For this review, take the finished solid that the model builds, in its own axes (mm). Face numbers are marked on the shaded views. A direction names the side the tool comes from. Coordinates: 2 decimals unless noted, no trailing zeros. Write each loop counter-clockwise with the first axis right and the second up, starting at its lowest first coordinate (ties: lowest second). Pieces come first, ordered by that corner, then holes. Notation, with made-up numbers: (-32, 7) - (-2, 7) arc R14 cw to (-2, 11) - close; hole circle Ø9 at (45, -32.5). An arc over 180 degrees is marked (long way). Use one line per item in the form item = value. Start each with the question number.
1) Tool access review of the marked faces 1, 2 and 3: name each direction out of +Z, -Z, +X, -X, +Y, -Y from which nothing blocks a thin tool from reaching the whole face with its end or side.
2) We need section C-C (y = 21.5). Give the boundary of the cut face in (x, z), plus the area to 3 significant figures.
3) We need section A-A (z = 3). Count the separate pieces of the cut face and the enclosed holes in it, plus the area to 3 significant figures.
4) For L1, parallel to Y at x = 23, z = 13.25; L2, parallel to Z at x = -52.5, y = -3, list the stretches that pass through material, from the lowest coordinate up. Write a range as from..to.
5) We need section B-B (x = -44.5). Give the boundary of the cut face in (y, z).
6) Insertion check: P1, Ø11.5, axis at x = 56, z = 9, coming from the -Y side; P2, Ø4.5, axis at x = -5.5, z = 6.5, coming from the +Y side; P3, Ø9.5, axis at y = 14, z = 7, coming from the -X side. Each pin has a flat end and moves straight along its axis. Give the tip position at first contact, or say it passes through.
```python
from build123d import *

# Parameters (mm, degrees)
F0_W     = 138
F0_H     = 55.5
F1_DEPTH = 1.5875
F2_W     = 14.4751365056
F2_H     = 21.9978075475
F3_DEPTH = 19


# Not quite as in the source:
# - a feature names something its author has since deleted; it is built from what else it names


with BuildPart() as f1:
    # F0 (on Top) → F1 (new body)
    with BuildSketch(Plane.XY):
        Rectangle(F0_W, F0_H)
    extrude(amount=F1_DEPTH)

    # F2 (on face) → F3 (join)
    with BuildSketch(Plane.XY.offset(1.5875)):
        with Locations((-25.527, 9.1310962263)):
            Rectangle(F2_W, F2_H)
        with Locations((-8.509, 9.1310962263)):
            Rectangle(F2_W, F2_H)
        with Locations((8.509, 9.1310962263)):
            Rectangle(F2_W, F2_H)
        with Locations((25.527, 9.1310962263)):
            Rectangle(F2_W, F2_H)
        with Locations((42.545, 9.1310962263)):
            Rectangle(F2_W, F2_H)
        with Locations((59.563, 9.1310962263)):
            Rectangle(F2_W, F2_H)
        with Locations((-42.545, 9.1310962263)):
            Rectangle(F2_W, F2_H)
        with Locations((-59.563, 9.1310962263)):
            Rectangle(F2_W, F2_H)
    extrude(amount=F3_DEPTH)


solid = f1.part
```
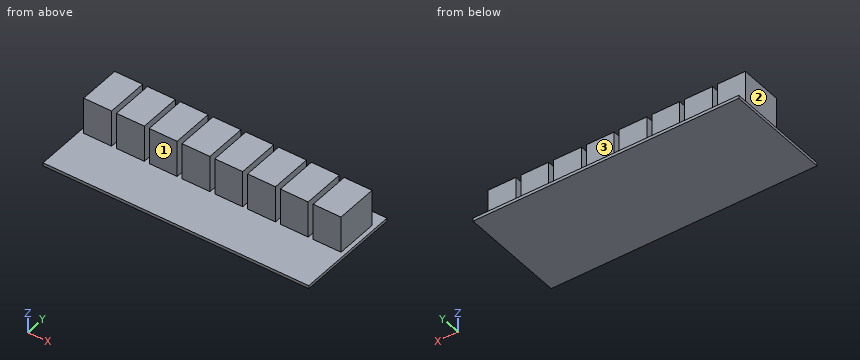
Determined:
q1.face_1 = +Z, +X, -X, -Y
q1.face_2 = +Z, -X, +Y, -Y
q1.face_3 = +Z, +X, -X, +Y
q2.outline = (-69, 0) - (69, 0) - (69, 1.59) - (-69, 1.59) - close
q2.area = 219 mm²
q3.separate_pieces = 8
q3.enclosed_holes = 0
q3.area = 2,550 mm²
q4.L1 = -1.87..20.13
q4.L2 = 0..1.59
q5.outline = (-27.75, 0) - (27.75, 0) - (27.75, 1.59) - (20.13, 1.59) - (20.13, 20.59) - (-1.87, 20.59) - (-1.87, 1.59) - (-27.75, 1.59) - close
q6.P1 = -1.87
q6.P2 = 20.13
q6.P3 = -66.8
